Geometry check sheet. Reference: the model listing, model coordinates, mm. Round coordinates to 2 decimals unless told otherwise and drop trailing zeros. Write each loop counter-clockwise with the first axis right and the second up, starting at its lowest first coordinate (ties: lowest second). Pieces come first, ordered by that corner, then holes. Notation, with made-up numbers: (35.25, 24) -> (75.25, 24) arc R18 ccw to (75.25, 59) -> close; hole circle Ø11 at (23, -39.5). An arc over 180 degrees is marked (long way). Put each result on its own line as item: value. Start each with the question number.
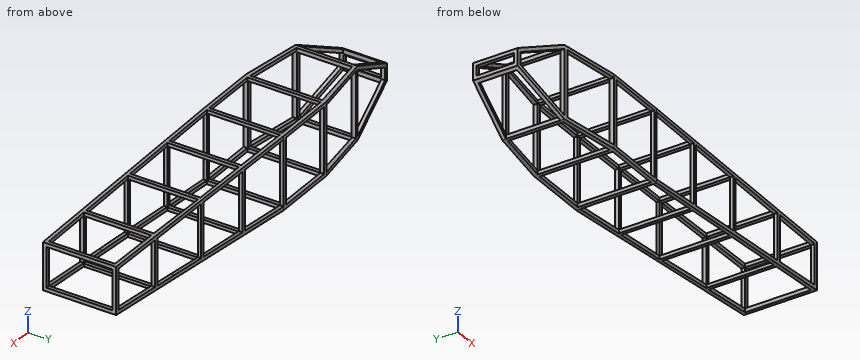
from build123d import *

# Parameters (mm, degrees)
F0_W      = 1524
F0_H      = 355.6
F2_DEPTH  = 127
F5_W      = 12.7
F5_H      = 295.684620738
F6_DEPTH  = 177.8
F8_DEPTH  = 190.5
F9_W      = 1716.6963219643
F9_H      = 471.6365635395
F10_DEPTH = 190.5
F12_DEPTH = 190.5
F13_W     = 1570.3657865524
F13_H     = 143.7467932701
F14_DEPTH = 190.5
F15_W     = 189.6323112059
F15_H     = 225.8323701404
F16_DEPTH = 25.4
F17_W     = 250.2110230158
F17_H     = 229.754279344
F18_DEPTH = 25.4
F19_W     = 254.0152243916
F19_H     = 229.5392287665
F20_DEPTH = 25.4
F21_W     = 248.717826187
F21_H     = 208.6506967284
F22_DEPTH = 25.4
F23_W     = 244.0285278141
F23_H     = 186.4718558426
F24_DEPTH = 15.24
F25_W     = 234.5546834328
F25_H     = 162.4008728846
F26_DEPTH = 13.97
F28_W     = 129.7433354616
F28_H     = 34.350046491
F29_DEPTH = 25.4
F30_W     = 228.6
F30_H     = 139.7
F31_DEPTH = 12.7


# Not quite as in the source:
# - a feature names something its author has since deleted; it is built from what else it names


with BuildPart() as f2:
    # F0 (on Top) → F2 (new body, symmetric)
    with BuildSketch(Plane.XY):
        Rectangle(F0_W, F0_H)
    extrude(amount=F2_DEPTH, both=True)

    # F5 (on Front) → F6 (join, symmetric)
    with BuildSketch(Plane.XZ):
        with Locations((-552.45, 4.7732368112)):
            Rectangle(F5_W, F5_H)
        with Locations((-336.55, 4.7732368112)):
            Rectangle(F5_W, F5_H)
        with Locations((-120.65, 4.7732368112)):
            Rectangle(F5_W, F5_H)
        with Locations((95.25, 4.7732368112)):
            Rectangle(F5_W, F5_H)
        with Locations((552.45, 4.7732368112)):
            Rectangle(F5_W, F5_H)
        with Locations((311.15, 4.7732368112)):
            Rectangle(F5_W, F5_H)
    extrude(amount=F6_DEPTH, both=True)

    # F7 (on Front) → F8 (cut, symmetric)
    with BuildSketch(Plane.XZ):
        Polygon((-1015.0121382617, 307.3465449898), (-843.425049348, -20.5651363992), (-558.8, 127), align=None)
        Polygon((-558.8, -127), (-762, -38.1), (-810.4430437088, -38.1), (-810.4430437088, -218.054279685), (819.7100162506, -218.054279685), (819.7100162506, -38.1), (762, -38.1), (-114.3, -127), align=None)
    extrude(amount=F8_DEPTH, both=True, mode=Mode.SUBTRACT)

    # F9 (on Top) → F10 (cut, symmetric)
    with BuildSketch(Plane.XY):
        with Locations((-0.0626146793, 9.3713402748)):
            Rectangle(F9_W, F9_H)
        Polygon((762, 127), (762, 0), (762, -127), (-114.3, -139.7), (-342.9, -139.7), (-762, -77.5716677308), (-762, 0), (-762, 77.5716677308), (-342.9, 139.7), (-114.3, 139.7), align=None, mode=Mode.SUBTRACT)
    extrude(amount=F10_DEPTH, both=True, mode=Mode.SUBTRACT)

    # F11 (on Top) → F12 (cut, symmetric)
    with BuildSketch(Plane.XY):
        Polygon((-749.2891273529, 66.8201254906), (-749.2891273529, -66.6171684709), (-558.8, -94.8557077165), (-558.8, 94.7766034894), align=None)
        Polygon((749.3002457909, -114.4827207254), (749.3002457909, 114.4827207254), (558.8, 117.2435938528), (558.8, -117.2435938528), align=None)
        Polygon((-127, -127.6207012333), (-127, 126.3945231583), (-330.2, 126.8815944692), (-330.2, -126.8815944692), align=None)
        Polygon((-546.1, -96.6881841261), (-342.9, -125.1055115079), (-342.9, 125.1055115079), (-546.1, 96.6881841261), align=None)
        Polygon((88.9, -124.4917157261), (88.9, 124.226110461), (-114.3, 126.3945231583), (-114.3, -127.4366432623), align=None)
        Polygon((101.6, 124.0527423648), (101.6, -124.3076577551), (304.8, -121.3627302188), (304.8, 122.6657975952), align=None)
        Polygon((317.5, 122.4924294991), (317.5, -120.8313876883), (546.1, -117.4366649156), (546.1, 117.1180185172), align=None)
    extrude(amount=F12_DEPTH, both=True, mode=Mode.SUBTRACT)

    # F13 (on Front) → F14 (cut, symmetric)
    with BuildSketch(Plane.XZ):
        Polygon((-558.8, 112.6946179402), (-749.3, 13.9290365255), (-749.3, -29.7940022002), (-558.8, -113.1377522002), align=None)
        Polygon((-546.1, -114.3), (-342.9, -114.3), (-342.9, 115.454279344), (-546.1, 115.7130942238), align=None)
        Polygon((558.8, -45.9493061315), (749.3, -26.623219175), (749.3, 114.3), (558.8, 114.3), align=None)
        Polygon((-330.2, -114.303525896), (-127, -114.3599402323), (-127, 115.1792885342), (-330.2, 115.438103414), align=None)
        Polygon((304.8, 114.6293069146), (101.6, 114.8881217944), (101.6, -92.4570416816), (304.8, -71.842548928), align=None)
        Polygon((456.2991908124, -56.4730658021), (546.1, -48.1008728846), (546.1, 114.3), (317.5, 114.6119749718), (317.5, -70.5541431309), align=None)
        with Locations((66.4489865303, 198.8733966351)):
            Rectangle(F13_W, F13_H)
        Polygon((-114.3, 115.1792885342), (-114.3, -114.3599402323), (88.9, -93.7454474787), (88.9, 114.9052492497), align=None)
    extrude(amount=F14_DEPTH, both=True, mode=Mode.SUBTRACT)

    # F15 (on face) → F16 (cut)
    with BuildSketch(Plane(origin=(-558.8, 0, 0), x_dir=(0, -1, 0), z_dir=(-1, 0, 0))):
        with Locations((0.0395521135, -0.22156713)):
            Rectangle(F15_W, F15_H)
    extrude(amount=-F16_DEPTH, mode=Mode.SUBTRACT)

    # F17 (on face) → F18 (cut)
    with BuildSketch(Plane(origin=(-342.9, 0, 0), x_dir=(0, -1, 0), z_dir=(-1, 0, 0))):
        with Locations((0, 0.577139672)):
            Rectangle(F17_W, F17_H)
    extrude(amount=-F18_DEPTH, mode=Mode.SUBTRACT)

    # F19 (on face) → F20 (cut)
    with BuildSketch(Plane(origin=(-127, 0, 0), x_dir=(0, -1, 0), z_dir=(-1, 0, 0))):
        with Locations((0.6130890375, 0.4096741509)):
            Rectangle(F19_W, F19_H)
    extrude(amount=-F20_DEPTH, mode=Mode.SUBTRACT)

    # F21 (on face) → F22 (cut)
    with BuildSketch(Plane(origin=(88.9, 0, 0), x_dir=(0, -1, 0), z_dir=(-1, 0, 0))):
        with Locations((0.1328026326, 10.5799008855)):
            Rectangle(F21_W, F21_H)
    extrude(amount=-F22_DEPTH, mode=Mode.SUBTRACT)

    # F23 (on face) → F24 (cut)
    with BuildSketch(Plane(origin=(304.8, 0, 0), x_dir=(0, -1, 0), z_dir=(-1, 0, 0))):
        with Locations((-0.6515336882, 21.3933789933)):
            Rectangle(F23_W, F23_H)
    extrude(amount=-F24_DEPTH, mode=Mode.SUBTRACT)

    # F25 (on face) → F26 (cut)
    with BuildSketch(Plane(origin=(546.1, 0, 0), x_dir=(0, -1, 0), z_dir=(-1, 0, 0))):
        with Locations((0.1593231992, 33.0995635577)):
            Rectangle(F25_W, F25_H)
    extrude(amount=-F26_DEPTH, mode=Mode.SUBTRACT)

    # F28 (on face) → F29 (cut)
    with BuildSketch(Plane(origin=(-762, 0, 0), x_dir=(0, -1, 0), z_dir=(-1, 0, 0))):
        with Locations((0, -8.2249767545)):
            Rectangle(F28_W, F28_H)
    extrude(amount=-F29_DEPTH, mode=Mode.SUBTRACT)

    # F30 (on face) → F31 (cut)
    with BuildSketch(Plane.YZ.offset(762)):
        with Locations((0, 44.45)):
            Rectangle(F30_W, F30_H)
    extrude(amount=-F31_DEPTH, mode=Mode.SUBTRACT)


solid = f2.part
(1) Material ranges on L1, parallel to X at y = 55, z = -31.5; L2, parallel to X at y = -102.5, z = -2; L3, parallel to Z at x = 684, y = 115.5, recorded low to high. Write a range as from..to.
(2) Sectioned sample at D-D (x = -522.5). Record the cut outline in (y, z), and give its area (3 significant figures).
(3) Sectioned sample at B-B (y = 16). State how many separate pieces and enclosed holes the cut face has, and give its area (3 significant figures).
(4) Go/stop test with flat-tipped pins: pin 1 Ø3 at (y, z) = (129, 17.5) entering from +X; pin 2 Ø4.5 at (y, z) = (-38.5, 119.5) entering from -X; pin 3 Ø4 at (y, z) = (-123.5, 50.5) entering from -X. Record where each tip stops, or that it passes through.
(5) Sectioned sample at A-A (x = 56). Record the cut outline in (y, z), and give its area (3 significant figures).
Found:
1. L1: -762..-749.29, 749.3..762
1. L2: -558.8..-546.1
1. L3: -46.01..-33.25, 114.3..127
2. outline: (-113.08, -127) -> (-99.99, -127) -> (-99.99, -114.3) -> (-113.08, -114.3) -> close; (-113.08, 115.68) -> (-99.99, 115.68) -> (-99.99, 127) -> (-113.08, 127) -> close; (99.99, -127) -> (113.08, -127) -> (113.08, -114.3) -> (99.99, -114.3) -> close; (99.99, 115.68) -> (113.08, 115.68) -> (113.08, 127) -> (99.99, 127) -> close
2. area: 629 mm2
3. separate pieces: 16
3. enclosed holes: 0
3. area: 2,630 mm2
4. pin 1: x = 558.8
4. pin 2: x = -558.8
4. pin 3: x = -342.9
5. outline: (-137.23, -109.72) -> (-124.97, -109.72) -> (-124.97, -97.08) -> (-137.23, -97.08) -> close; (-137.23, 114.95) -> (-124.97, 114.95) -> (-124.97, 127) -> (-137.23, 127) -> close; (124.58, -109.72) -> (137.23, -109.72) -> (137.23, -97.08) -> (124.58, -97.08) -> close; (124.58, 114.95) -> (137.23, 114.95) -> (137.23, 127) -> (124.58, 127) -> close
5. area: 615 mm2
